Geometry check sheet. Reference: the model listing, model coordinates, mm. Face numbers are marked on the shaded views. A direction names the side the tool comes from. Give positions to 0.01 mm unless a question says otherwise; leave off trailing zeros. Write each loop counter-clockwise with the first axis right and the second up, starting at its lowest first coordinate (ties: lowest second). Pieces come first, ordered by that corner, then holes. Notation, with made-up numbers: (7.25, -39.5) -> (48.25, -39.5) arc R19 cw to (48.25, -8.5) -> close; hole circle Ø3 at (67, 60.5). An arc over 180 degrees is marked (long way). One line per item, written item: value.
from build123d import *

# Parameters (mm, degrees)
F0_R     = 21.4314801072
F1_DEPTH = 12.7
F2_R     = 5.08
F3_T     = -2.54


# Not quite as in the source:
# - a shell that OpenCascade refuses in one call is made with other operations: the cavity is built on its own and cut out


with BuildPart() as f1:
    # F0 (on Front) → F1 (new body, symmetric)
    with BuildSketch(Plane.XZ):
        with BuildLine():
            Line((0, 102.3351529121), (0, 0))
            Line((0, 0), (99.1575824261, 0))
            ThreePointArc((99.1575824261, 0), (117.1180946682, 7.4394877579), (124.5575824261, 25.4))
            Line((124.5575824261, 25.4), (124.5575824261, 95.9851529121))
            ThreePointArc((124.5575824261, 95.9851529121), (122.6977104866, 100.4752809727), (118.2075824261, 102.3351529121))
            Line((118.2075824261, 102.3351529121), (0, 102.3351529121))
        make_face()
        with Locations((37.157318583, 35.142709024)):
            Circle(F0_R, mode=Mode.SUBTRACT)
    extrude(amount=F1_DEPTH, both=True)

    # F2
    f2_edges = [f1.edges().sort_by_distance(p)[0] for p in [
        (59.103791, 12.7, 102.335153),
        (59.103791, -12.7, 102.335153),
    ]]
    fillet(f2_edges, radius=F2_R)

    # F3: a shell. OpenCascade refuses it in one call, so the cavity is built on its own and cut out:
    # the body offset inwards by the wall thickness, plus a prism from it out through each open face.
    f3_core = offset(f1.part, amount=F3_T, mode=Mode.PRIVATE)
    f3_exits = [f3_core.faces().sort_by_distance(p)[0] for p in [
        (65.31507, -10.16, 54.836293),
    ]]
    add(f3_core, mode=Mode.SUBTRACT)
    extrude(f3_exits, amount=-F3_T, mode=Mode.SUBTRACT)


solid = f1.part
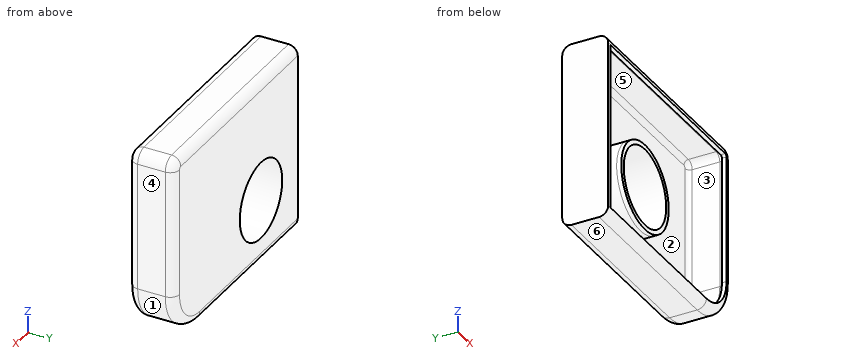
1) Sectioned sample at A-A on y = -4.5. Record the cut outline in (x, z), plus the area to 3 significant figures.
Verdict:
outline: (0, 0) -> (99.16, 0) arc R25.4 ccw to (124.56, 25.4) -> (124.56, 95.99) arc R6.35 ccw to (118.21, 102.34) -> (0, 102.34) -> close; circle Ø47.94 at (37.16, 35.14); hole (2.54, 2.54) -> (99.16, 2.54) arc R22.86 ccw to (122.02, 25.4) -> (122.02, 95.99) arc R3.81 ccw to (118.21, 99.8) -> (2.54, 99.8) -> close; hole circle Ø42.86 at (37.16, 35.14)
area: 1,460 mm^2
2) Sectioned sample at C-C on z = 28. Record the cut outline in (x, y), plus the area to 3 significant figures.
Verdict:
outline: (0, -12.7) -> (2.54, -12.7) -> (2.54, 10.16) -> (14.27, 10.16) -> (14.27, -12.7) -> (16.95, -12.7) -> (16.95, 12.7) -> (0, 12.7) -> close; (57.36, -12.7) -> (60.04, -12.7) -> (60.04, 10.16) -> (119.48, 10.16) arc R2.54 cw to (122.02, 7.62) -> (122.02, -7.62) arc R2.54 cw to (119.48, -10.16) -> (119.48, -12.7) arc R5.08 ccw to (124.56, -7.62) -> (124.56, 7.62) arc R5.08 ccw to (119.48, 12.7) -> (57.36, 12.7) -> close
area: 450 mm^2
3) Depth check by flat-ended pin: pin 1 Ø2 at (x, y) = (85, -11) entering from -Z; pin 2 Ø6 at (x, z) = (53, 84) entering from -Y; pin 3 Ø0.8 at (x, y) = (30.5, -11) entering from +Z. Enter the tip coordinate at first touch or a pass-through.
Verdict:
pin 1: z = 0.59
pin 2: y = 10.16
pin 3: z = 101.37
4) Sectioned sample at B-B on x = 56. Record the cut outline in (y, z).
Verdict:
outline: (-12.7, 5.08) arc R5.08 ccw to (-7.62, 0) -> (7.62, 0) arc R5.08 ccw to (12.7, 5.08) -> (12.7, 24.93) -> (-12.7, 24.93) -> (-12.7, 20.32) -> (10.16, 20.32) -> (10.16, 5.08) arc R2.54 cw to (7.62, 2.54) -> (-7.62, 2.54) arc R2.54 cw to (-10.16, 5.08) -> close; (-12.7, 45.35) -> (12.7, 45.35) -> (12.7, 97.26) arc R5.08 ccw to (7.62, 102.34) -> (-7.62, 102.34) arc R5.08 ccw to (-12.7, 97.26) -> (-10.16, 97.26) arc R2.54 cw to (-7.62, 99.8) -> (7.62, 99.8) arc R2.54 cw to (10.16, 97.26) -> (10.16, 49.96) -> (-12.7, 49.96) -> close
5) Sectioned sample at D-D on z = 65. Record the cut outline in (x, y), plus the area to 3 significant figures.
Verdict:
outline: (0, -12.7) -> (2.54, -12.7) -> (2.54, 10.16) -> (119.48, 10.16) arc R2.54 cw to (122.02, 7.62) -> (122.02, -7.62) arc R2.54 cw to (119.48, -10.16) -> (119.48, -12.7) arc R5.08 ccw to (124.56, -7.62) -> (124.56, 7.62) arc R5.08 ccw to (119.48, 12.7) -> (0, 12.7) -> close
area: 431 mm^2
6) Scan lines: probe 1 along Z at (x, y) = (88, -0.25); probe 2 along X at (y, z) = (-1, 47); probe 3 along Z at (x, y) = (25, -8). Record each from-to range of solid material in increasing order.
Verdict:
probe 1: 0 to 2.54, 99.8 to 102.34
probe 2: 0 to 2.54, 16.32 to 19.3, 55.01 to 57.99, 122.02 to 124.56
probe 3: 0.01 to 2.57, 14.48 to 17.49, 52.79 to 55.8, 99.77 to 102.32
7) Tool access check on the marked faces 5 and 6. Record the directions out of +Z, -Z, +X, -X, +Y, -Y that give a thin tool (end or side, any length) a straight path to the whole face; none if there is none.
Verdict:
face 5: none
face 6: -Z, +X, -X, +Y, -Y
8) Mould release check, pull along Z, two halves, no side actions. Record for the marked faces 1, 2, 3 and 4: released by +Z, released by -Z, zero draft, split by the parting line, or undercut.
Verdict:
face 1: released by -Z
face 2: undercut
face 3: undercut
face 4: zero draft
